Geometry: see drawing. Coordinates: mm, zero at the bounding-box minimum. A direction names the side the tool comes from. Round coordinates to 2 decimals unless told otherwise and drop trailing zeros. Loops run counter-clockwise (first coordinate to the right, second up) from the corner with the lowest first, then second, coordinate; pieces in that order, holes last.
(1) Cut plane A-A, the plane y = 8.5. Output: boundary loops of the cut face in (x, z), and give its area (3 significant figures).
(2) Cut plane C-C, the plane z = 0.8. Output: boundary loops of the cut face in (x, y), and give its area (3 significant figures).
(3) First-contact query: pin 1 Ø5 at (x, y) = (14.5, 7) entering from -Z; pin 2 Ø3 at (y, z) = (8.5, 2) entering from +X. Flat tips, straight axial feed; report the tip coordinate or a pass-through.
(4) Line query: line 1 (Y direction, x = 8.5, z = 3.4); line 2 (Z direction, x = 7.25, y = 1); line 3 (Y direction, x = 9, z = 4.25). Output: solid intervals per line, ascending.
(5) Access query for the marked faces 1 and 2. Directions: +Z, -Z, +X, -X, +Y, -Y. A direction counts if a zero-diameter tool reaches every point of the face in a straight line with its end or side. Return the directions, or none.
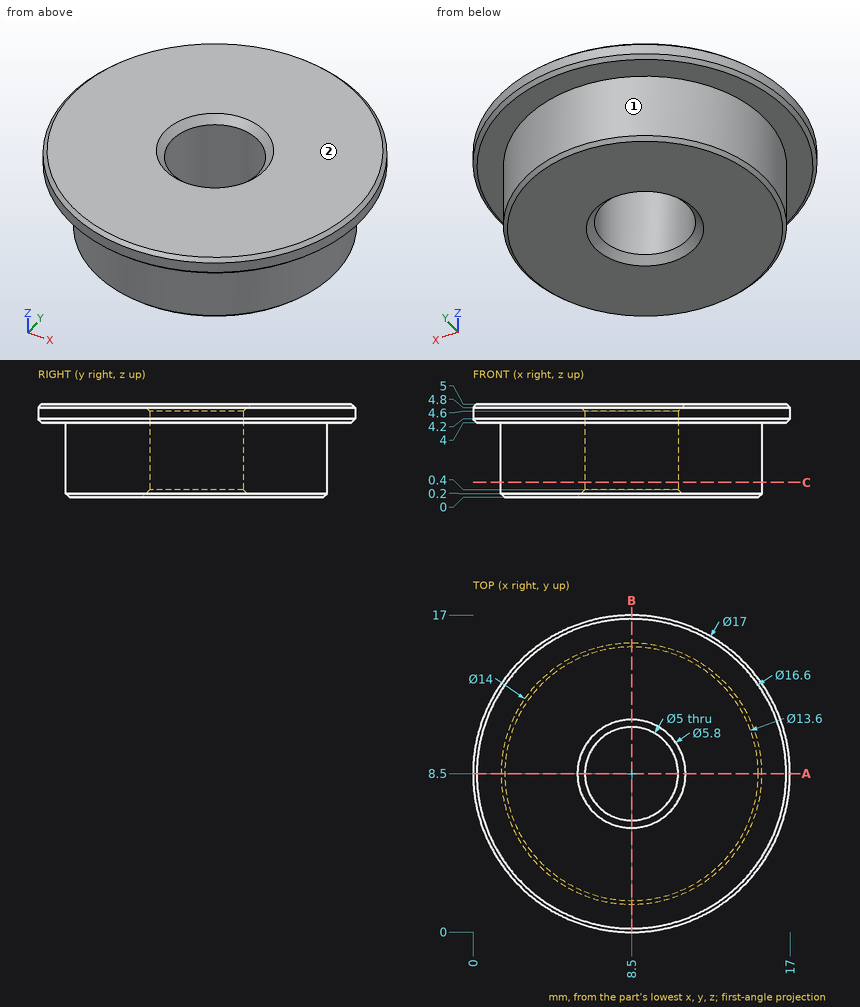
Reported:
1. outline: (0, 4.2) - (0.2, 4) - (1.5, 4) - (1.5, 0.2) - (1.7, 0) - (5.6, 0) - (6, 0.4) - (6, 4.6) - (5.6, 5) - (0.2, 5) - (0, 4.8) - close; (11, 0.4) - (11.4, 0) - (15.3, 0) - (15.5, 0.2) - (15.5, 4) - (16.8, 4) - (17, 4.2) - (17, 4.8) - (16.8, 5) - (11.4, 5) - (11, 4.6) - close
1. area: 47.6 mm2
2. outline: circle Ø14 at (8.5, 8.5); hole circle Ø5 at (8.5, 8.5)
2. area: 134 mm2
3. pin 1: stops at z = 0
3. pin 2: stops at x = 15.5
4. line 1: y = 1.5 to 6, 11 to 15.5
4. line 2: z = 4 to 5
4. line 3: y = 0.01 to 6.05, 10.95 to 16.99
5. face 1: -Z
5. face 2: +Z, +X, -X, +Y, -Y
